```python
from build123d import *

# Parameters (mm, degrees)
EXTRUDE_1_DEPTH     = 23
CUT_EXTRUDE_START   = 3.25
SKETCH_2_R          = 1
CUT_EXTRUDE_1_DEPTH = 3


with BuildPart() as part:
    # 草图1 → 凸台-拉伸1 (new body)
    with BuildSketch(Plane.XY):
        Polygon((3.5, -1.85), (3.5, -3.25), (8.5, -3.25), (8.5, 3.25), (-8.5, 3.25), (-8.5, -3.25), (-3.5, -3.25), (-3.5, -1.85), (-2.5, -1.85), (-2.5, -1.1), (-3.5, -1.1), (-3.5, 0.25), (3.5, 0.25), (3.5, -1.1), (2.5, -1.1), (2.5, -1.85), align=None)
    extrude(amount=EXTRUDE_1_DEPTH)

    # 草图2 → 切除-拉伸1 (cut)
    with BuildSketch(Plane(origin=(0, 0, 0), x_dir=(1, 0, 0), z_dir=(0, 1, 0)).offset(CUT_EXTRUDE_START)):
        with Locations((-6, -7)):
            Circle(SKETCH_2_R)
        with Locations((6, -7)):
            Circle(SKETCH_2_R)
        with Locations((-6, -15)):
            Circle(SKETCH_2_R)
        with Locations((6, -15)):
            Circle(SKETCH_2_R)
    extrude(amount=-CUT_EXTRUDE_1_DEPTH, mode=Mode.SUBTRACT)


solid = part.part
```
Input: part model. Units: mm. Frame: model coordinates. A direction names the side the tool comes from. Give positions to 0.01 mm unless a question says otherwise; leave off trailing zeros. Loops run counter-clockwise (first coordinate to the right, second up) from the corner with the lowest first, then second, coordinate; pieces in that order, holes last. Notation, with made-up numbers: M -18,28.25 L 10,28.25 A14 ccw 10,51.25 Z; hole C 72,-16.5 d5. An arc over 180 degrees is marked long. Answer as CSV lines item,"result". Start each with the question number.
1. Reachability of faces 1 (the face through (-3.5, -3, 11)), 2 (the face through (-6, 0.25, 15)), 3 (the face through (3, -1.1, 11)) from +Z, -Z, +X, -X, +Y, -Y: full face, straight path, thin tool, end or side. Return the list, or none.
2. Section A-A on y = 0. Return loops of the section in (x, z).
3. Section C-C on z = 13.5. Return loops of the section in (x, y), plus the area to 3 significant figures.
4. Pin query (flat end, axial travel): P1, Ø1, axis at x = -0.5, z = 9.5, coming from the -Y side; P2, Ø2, axis at x = 6.5, z = 15, coming from the +Y side; P3, Ø1.6, axis at x = -6, z = 7, coming from the +Y side; P4, Ø0.8, axis at x = -3, z = 16.5, coming from the -Y side. Return the tip coordinate at first contact, or that it passes through.
5. Section D-D on z = 7. Return loops of the section in (x, y), plus the area to 3 significant figures.
6. Section B-B on x = 6. Return loops of the section in (y, z).
7. Line query: L1, parallel to Z at x = -6, y = 2.3; L2, parallel to X at y = 1.35, z = 7; L3, parallel to Y at x = 2.75, z = 20.25. Output: solid intervals per line, ascending.
8. Pull-direction query (Y, two-part tool) for faces 4 (the face through (-3, -1.1, 11)), 5 (the face through (0, 0.25, 11)), 6 (the face through (0, 3.25, 11)), 7 (the face through (5.263, 1.771, 6.324)); classes: released by +Y, released by -Y, zero draft, split by the parting line, or undercut.
Computed values:
1,face 1,"+Z, -Z, -Y"
1,face 2,"+Y"
1,face 3,"+Z, -Z"
2,outline,"M -8.5,0 L -3.5,0 L -3.5,23 L -8.5,23 Z; M 3.5,0 L 8.5,0 L 8.5,23 L 3.5,23 Z"
3,outline,"M -8.5,-3.25 L -3.5,-3.25 L -3.5,-1.85 L -2.5,-1.85 L -2.5,-1.1 L -3.5,-1.1 L -3.5,0.25 L 3.5,0.25 L 3.5,-1.1 L 2.5,-1.1 L 2.5,-1.85 L 3.5,-1.85 L 3.5,-3.25 L 8.5,-3.25 L 8.5,3.25 L -8.5,3.25 Z"
3,area,"87.5 mm²"
4,P1,"stops at y = 0.25"
4,P2,"stops at y = 3.25"
4,P3,"stops at y = 0.25"
4,P4,"stops at y = -1.85"
5,outline,"M -8.5,-3.25 L -3.5,-3.25 L -3.5,-1.85 L -2.5,-1.85 L -2.5,-1.1 L -3.5,-1.1 L -3.5,0.25 L 3.5,0.25 L 3.5,-1.1 L 2.5,-1.1 L 2.5,-1.85 L 3.5,-1.85 L 3.5,-3.25 L 8.5,-3.25 L 8.5,3.25 L 7,3.25 L 7,0.25 L 5,0.25 L 5,3.25 L -5,3.25 L -5,0.25 L -7,0.25 L -7,3.25 L -8.5,3.25 Z"
5,area,"75.5 mm²"
6,outline,"M -3.25,0 L 3.25,0 L 3.25,6 L 0.25,6 L 0.25,8 L 3.25,8 L 3.25,14 L 0.25,14 L 0.25,16 L 3.25,16 L 3.25,23 L -3.25,23 Z"
7,L1,"z = 0 to 6, 8 to 14, 16 to 23"
7,L2,"x = -8.5 to -7, -5 to 5, 7 to 8.5"
7,L3,"y = -1.85 to -1.1, 0.25 to 3.25"
8,face 4,"undercut"
8,face 5,"undercut"
8,face 6,"released by +Y"
8,face 7,"zero draft"
